Work out the finished part from the listing and answer in its coordinate system (mm). Face numbers are marked on the shaded views. A direction names the side the tool comes from. Round coordinates to 2 decimals unless told otherwise and drop trailing zeros. Write each loop counter-clockwise with the first axis right and the second up, starting at its lowest first coordinate (ties: lowest second). Pieces come first, ordered by that corner, then holes. Notation, with made-up numbers: M 82.25,29.25 L 93.25,29.25 A6 cw 93.25,36.25 Z; hole C 66.5,85 d8. An arc over 180 degrees is marked long. Answer in a Markdown table with one row per item.
```python
from build123d import *

# Parameters (mm, degrees)
F1_DEPTH  = 3
F3_DEPTH  = 2
F4_R      = 1.5
F5_DEPTH  = 3
F6_SIZE   = 1
F7_R      = 1
F9_DEPTH  = 1.0010001
F10_R     = 1.49999
F11_W     = 6
F11_H     = 1.5
F12_DEPTH = 2.5


# Not quite as in the source:
# - a fillet or chamfer is up to 0.001 mm smaller than in the source, because OpenCascade refuses the exact size


with BuildPart() as f1:
    # F0 (on Top) → F1 (new body)
    with BuildSketch(Plane.XY):
        with BuildLine():
            Line((-4, 20), (-4, 14.4568322948))
            ThreePointArc((-4, 14.4568322948), (0, -15), (4, 14.4568322948))
            Line((4, 14.4568322948), (4, 20))
            Line((4, 20), (-4, 20))
        make_face()
    extrude(amount=F1_DEPTH)

    # F2 (on face) → F3 (cut)
    with BuildSketch(Plane.XY.offset(3)):
        with BuildLine():
            Line((1.5, 20), (-1.5, 20))
            Line((-1.5, 20), (-1.5, 10.3923048454))
            ThreePointArc((-1.5, 10.3923048454), (0, -10.5), (1.5, 10.3923048454))
            Line((1.5, 10.3923048454), (1.5, 20))
        make_face()
    extrude(amount=-F3_DEPTH, mode=Mode.SUBTRACT)

    # F4 (on face) → F5 (join)
    with BuildSketch(Plane.XY.offset(3)):
        with Locations((12.5, 0)):
            Circle(F4_R)
        with Locations((-12.5, 0)):
            Circle(F4_R)
        with Locations((0, -12.5)):
            Circle(F4_R)
    extrude(amount=F5_DEPTH)

    # F6
    f6_edges = [f1.edges().sort_by_distance(p)[0] for p in [
        (-14, 0, 6),
        (-1.5, -12.5, 6),
        (11, 0, 6),
    ]]
    chamfer(f6_edges, length=F6_SIZE)

    # F7
    f7_edges = [f1.edges().sort_by_distance(p)[0] for p in [
        (4, 17.228416, 0),
        (4, 14.456832, 1.5),
        (-4, 14.456832, 1.5),
        (-4, 17.228416, 0),
        (0, -15, 0),
    ]]
    fillet(f7_edges, radius=F7_R)

    # F8 (on face) → F9 (cut, through all)
    with BuildSketch(Plane.XY.offset(1)):
        with BuildLine():
            Line((-1.5, 9.633924434), (-1.5, 9.8868599666))
            ThreePointArc((-1.5, 9.8868599666), (0, -10), (1.5, 9.8868599666))
            Line((1.5, 9.8868599666), (1.5, 9.633924434))
            ThreePointArc((1.5, 9.633924434), (0, -9.75), (-1.5, 9.633924434))
        make_face()
    extrude(amount=-F9_DEPTH, mode=Mode.SUBTRACT)

    # F10 (radius 1.5 in the source; OpenCascade refuses exactly that, so slightly less here)
    f10_edges = [f1.edges().sort_by_distance(p)[0] for p in [
        (1.5, 15.196152, 1),
        (-1.5, 15.196152, 1),
    ]]
    fillet(f10_edges, radius=F10_R)

    # F11 (on face) → F12 (cut)
    with BuildSketch(Plane.XY.offset(3)):
        with Locations((0, 14.75)):
            Rectangle(F11_W, F11_H)
    extrude(amount=-F12_DEPTH, mode=Mode.SUBTRACT)


solid = f1.part
```
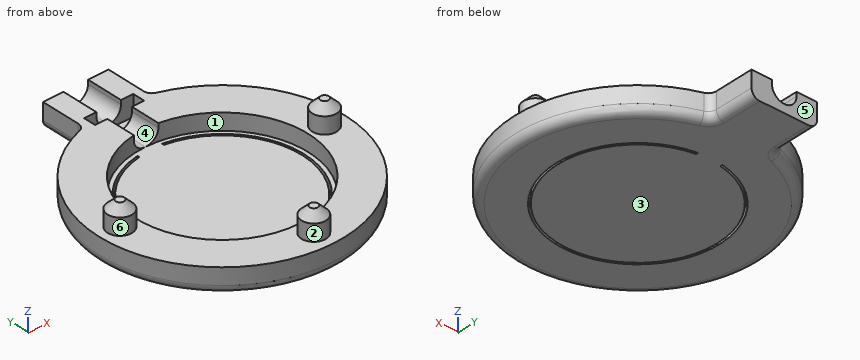
1. Determine the mould class of the marked faces 1, 2 and 3 for opening direction Y: released by +Y, released by -Y, zero draft, split by the parting line, or undercut.
Calculated:
| item | result |
|---|---|
| face 1 | undercut |
| face 2 | split by the parting line |
| face 3 | zero draft |
2. The part is cut by section A-A (z = 4.25). Determine the outline of the cut face in (x, y), plus the area to 3 significant figures.
Calculated:
| item | result |
|---|---|
| outline | C -12.5,0 d3; C 0,-12.5 d3; C 12.5,0 d3 |
| area | 21.2 mm² |
3. The part is cut by section B-B (y = 0). Count the separate pieces of the cut face and the enclosed holes in it, plus the area to 3 significant figures.
Calculated:
| item | result |
|---|---|
| separate pieces | 3 |
| enclosed holes | 0 |
| area | 63.1 mm² |
4. A tool of negligible diameter and unlimited length cuts with its end or side. For the marked faces 4, 5 and 6, from which of +Z, -Z, +X, -X, +Y, -Y can it reach the whole face along a straight path? Write none if from no direction.
Calculated:
| item | result |
|---|---|
| face 4 | +Z, +Y |
| face 5 | +Z, -Z, +X, -X, +Y |
| face 6 | +Z |
5. The part is cut by section C-C (z = 2). Determine the outline of the cut face in (x, y).
Calculated:
| item | result |
|---|---|
| outline | M -4.69,14.25 A15 ccw long 4.69,14.25 A1 cw 4,15.2 L 4,20 L 1.41,20 L 1.41,15.5 L 3,15.5 L 3,14 L 1.41,14 L 1.41,10.4 A10.5 cw long -1.41,10.4 L -1.41,14 L -3,14 L -3,15.5 L -1.41,15.5 L -1.41,20 L -4,20 L -4,15.2 A1 cw Z |
6. Consider line 1 along X through (y, z) = (0, 0.3); line 2 along X through (y, z) = (0, 2.2); line 3 along X through (y, z) = (0, 0.4). Determine where each line is inside the solid, lowest interval first. Write a range as from..to.
Calculated:
| item | result |
|---|---|
| line 1 | x = -14.71..-10, -9.75..9.75, 10..14.71 |
| line 2 | x = -15..-10.5, 10.5..15 |
| line 3 | x = -14.8..-10, -9.75..9.75, 10..14.8 |
7. Given pin 1 (1 mm diameter, centred on x = -3.5, y = -4.5, fed in from +Z); pin 2 (10 mm diameter, centred on x = 7.5, y = 13.5, fed in from +Z); pin 3 (0.6 mm diameter, centred on y = 17, z = 2.5, fed in from -X); pin 4 (2 mm diameter, centred on y = -9.5, z = 4.5, fed in from -X), each flat-ended and moving along its own axis, determine where each tip first touches the part or whether it passes through.
Calculated:
| item | result |
|---|---|
| pin 1 | stops at z = 1 |
| pin 2 | stops at z = 3 |
| pin 3 | stops at x = -4 |
| pin 4 | passes through |
